from build123d import *

# Parameters (mm, degrees)
F0_W     = 65
F0_H     = 38
F1_DEPTH = 35
F2_W     = 62
F2_H     = 34
F3_DEPTH = 32.5
F4_R     = 2.75
F5_DEPTH = 8
F7_DEPTH = 36


with BuildPart() as f1:
    # F0 (on Top) → F1 (new body)
    with BuildSketch(Plane.XY):
        Rectangle(F0_W, F0_H)
    extrude(amount=F1_DEPTH)

    # F2 (on face) → F3 (cut)
    with BuildSketch(Plane.XY.offset(35)):
        Rectangle(F2_W, F2_H)
    extrude(amount=-F3_DEPTH, mode=Mode.SUBTRACT)

    # F4 (on face) → F5 (join)
    with BuildSketch(Plane.XZ.offset(19)):
        with Locations((-12.5, 5)):
            Circle(F4_R)
        with Locations((-12.5, 30)):
            Circle(F4_R)
        with Locations((12.5, 30)):
            Circle(F4_R)
        with Locations((12.5, 5)):
            Circle(F4_R)
    extrude(amount=F5_DEPTH)

    # F6 (on face) → F7 (cut, through all)
    with BuildSketch(Plane(origin=(0, 19, 0), x_dir=(-1, 0, 0), z_dir=(0, 1, 0))):
        Polygon((32.5, 35), (-32.5, 35), (0, 10), align=None)
    extrude(amount=-F7_DEPTH, mode=Mode.SUBTRACT)


solid = f1.part
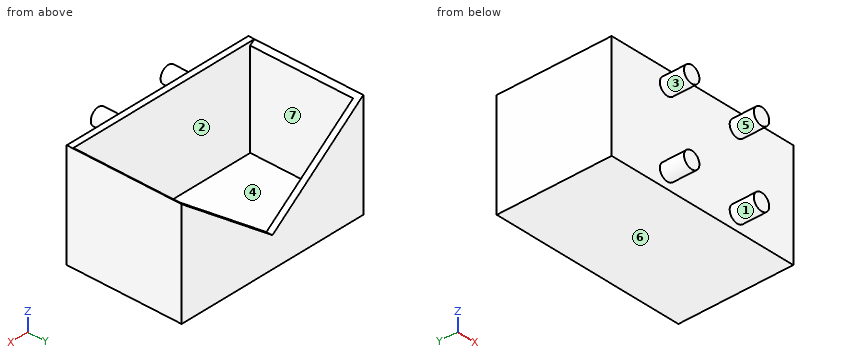
Verification items for the finished model (mm, model axes). Face numbers are marked on the shaded views. A direction names the side the tool comes from. Give positions to 0.01 mm unless a question says otherwise; leave off trailing zeros. Loops run counter-clockwise (first coordinate to the right, second up) from the corner with the lowest first, then second, coordinate; pieces in that order, holes last.
1) Sectioned sample at C-C, the plane y = 13. Enter the section's corners in (x, z).
2) Thickness scan on line 1 along Y through (x, z) = (25.5, 14); line 2 along X through (y, z) = (-7, 14); line 3 along Z through (x, y) = (-17.5, 12). Record the ranges inside material, lowest first.
3) Set-up check for the marked faces 5, 6 and 7: record each of +Z, -Z, +X, -X, +Y, -Y from which the full face is reachable in a straight line by a thin tool's end or side.
4) Sectioned sample at A-A, the plane z = 5. Enter the section's corners in (x, y).
5) Depth check by flat-ended pin: pin 1 Ø1 at (x, y) = (10.5, -6) entering from +Z; pin 2 Ø4 at (x, z) = (-1.5, 19) entering from -Y. Enter the tip coordinate at first touch or a pass-through.
6) Sectioned sample at D-D, the plane x = 1.5. Enter the section's corners in (y, z), then the cut area to 3 significant figures.
7) Sectioned sample at B-B, the plane z = 30. Enter the section's corners in (x, y).
8) Draft check along Z on the marked faces 1, 2, 3 and 4. Enter one of: pulls with the +Z half, pulls with the -Z half, needs draft (parallel to the pull), parting line crosses it, or undercut.
Answers:
1. outline: (-32.5, 0) - (32.5, 0) - (32.5, 35) - (31, 33.85) - (31, 2.5) - (-31, 2.5) - (-31, 33.85) - (-32.5, 35) - close
2. line 1: y = -19 to -17, 17 to 19
2. line 2: x = -32.5 to -31, 31 to 32.5
2. line 3: z = 0 to 2.5
3. face 5: -Y
3. face 6: -Z, +X, -X, +Y, -Y
3. face 7: +Z
4. outline: (-32.5, -19) - (-15.25, -19) - (-15.25, -27) - (-9.75, -27) - (-9.75, -19) - (9.75, -19) - (9.75, -27) - (15.25, -27) - (15.25, -19) - (32.5, -19) - (32.5, 19) - (-32.5, 19) - close; hole (-31, -17) - (31, -17) - (31, 17) - (-31, 17) - close
5. pin 1: stops at z = 2.5
5. pin 2: stops at y = -19
6. outline: (-19, 0) - (19, 0) - (19, 11.15) - (17, 11.15) - (17, 2.5) - (-17, 2.5) - (-17, 35) - (-19, 35) - close
6. area: 177 mm2
7. outline: (-32.5, -19) - (-15.25, -19) - (-15.25, -27) - (-9.75, -27) - (-9.75, -19) - (9.75, -19) - (9.75, -27) - (15.25, -27) - (15.25, -19) - (32.5, -19) - (32.5, 19) - (26, 19) - (26, 17) - (31, 17) - (31, -17) - (-31, -17) - (-31, 17) - (-26, 17) - (-26, 19) - (-32.5, 19) - close
8. face 1: undercut
8. face 2: needs draft
8. face 3: undercut
8. face 4: pulls with the +Z half
